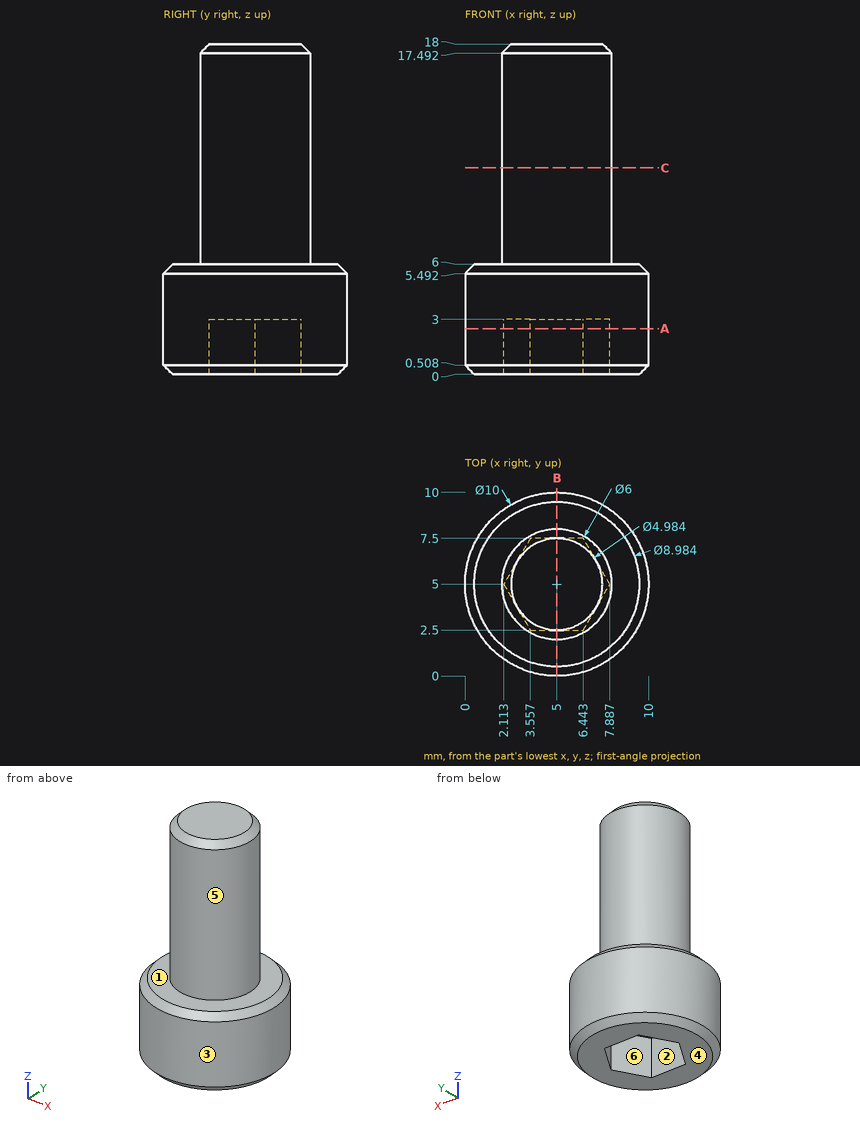
The figure shows three views and two pictorial views of one solid part (mm, origin at its lowest corner). Answer the questions. A direction names the side the tool comes from. Round coordinates to 2 decimals unless told otherwise and drop trailing zeros. Write each loop counter-clockwise with the first axis right and the second up, starting at its lowest first coordinate (ties: lowest second). Pieces come first, ordered by that corner, then holes. Notation, with made-up numbers: M 3,65.5 L 18,65.5 A29 cw 18,104.5 Z; hole C -17,58 d11. An arc over 180 degrees is marked long. Use a Markdown table: item, result.
1) The part is cut by section C-C (z = 11.25). Write down the section's boundary in (x, y).
Answers follow:
| item | result |
|---|---|
| outline | C 5,5 d6 |
2) Straight lines are drawn through the part: line 1 along Z through (x, y) = (5, 7.25); line 2 along Z through (x, y) = (3, 2.5); line 3 along Y through (x, z) = (3, 1.5) (1 decimal). For each, find the intervals that lie inside material, in ascending order. Write a range as [from, to].
Answers follow:
| item | result |
|---|---|
| line 1 | z = [3, 18] |
| line 2 | z = [0, 6] |
| line 3 | y = [0.4, 3.5], [6.5, 9.6] |
3) For a pull along Y with two mould halves and no side action, classify the marked faces 1, 2 and 3 as pulls with the +Y half, pulls with the -Y half, needs draft (parallel to the pull), parting line crosses it, or undercut.
Answers follow:
| item | result |
|---|---|
| face 1 | needs draft |
| face 2 | undercut |
| face 3 | parting line crosses it |
4) A tool of negligible diameter and unlimited length cuts with its end or side. For the marked faces 4, 5 and 6, from which of +Z, -Z, +X, -X, +Y, -Y can it reach the whole face along a straight path? Write none if from no direction.
Answers follow:
| item | result |
|---|---|
| face 4 | -Z, +X, -X, +Y, -Y |
| face 5 | +Z |
| face 6 | -Z |
5) The part is cut by section A-A (z = 2.5). Write down the section's boundary in (x, y).
Answers follow:
| item | result |
|---|---|
| outline | C 5,5 d10; hole M 2.11,5 L 3.56,2.5 L 6.44,2.5 L 7.89,5 L 6.44,7.5 L 3.56,7.5 Z |
6) Flat-ended cylindrical pins translate along their axes: pin 1 (1.5 mm diameter, centred on x = 5.5, y = 4.5, fed in from -Z); pin 2 (6 mm diameter, centred on x = 5.5, z = 10, fed in from +Y); pin 3 (3 mm diameter, centred on y = 7.5, z = 2, fed in from +X). Find the tip coordinate at first contact, or state that the pin passes through.
Answers follow:
| item | result |
|---|---|
| pin 1 | stops at z = 3 |
| pin 2 | stops at y = 8 |
| pin 3 | stops at x = 9.9 |
7) The part is cut by section B-B (x = 5). Write down the section's boundary in (y, z), plus the area to 3 significant figures.
Answers follow:
| item | result |
|---|---|
| outline | M 0,0.51 L 0.51,0 L 2.5,0 L 2.5,3 L 7.5,3 L 7.5,0 L 9.49,0 L 10,0.51 L 10,5.49 L 9.49,6 L 8,6 L 8,17.49 L 7.49,18 L 2.51,18 L 2,17.49 L 2,6 L 0.51,6 L 0,5.49 Z |
| area | 116 mm2 |
